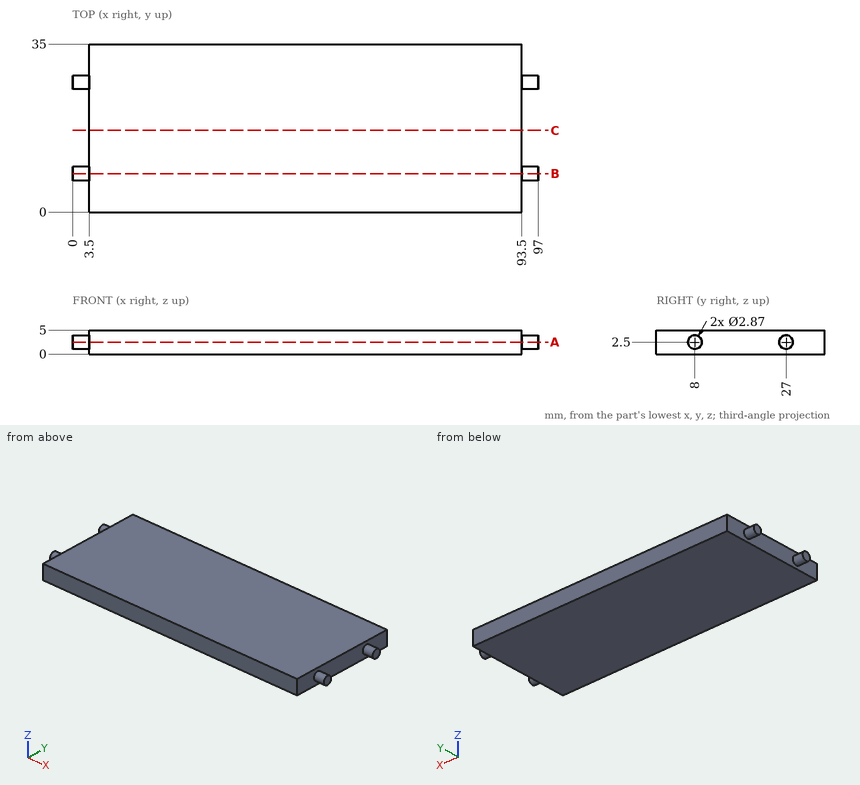
Geometry check sheet. Reference: drawing and pictorial views, mm from the part's lowest x, y, z. Give positions to 0.01 mm unless a question says otherwise; leave off trailing zeros. Write each loop counter-clockwise with the first axis right and the second up, starting at its lowest first coordinate (ties: lowest second). Pieces come first, ordered by that corner, then holes.
Item 1: Scan line: L1, parallel to X at y = 4, z = 2.2. Record every from-to range of solid material in increasing order.
Item 2: Cross-section at C-C (y = 17). Enter the section's corners in (x, z), and give its area (3 significant figures).
Item 3: Gauge pin test, flat ends, axial feed: pin 1 (3 mm diameter, centred on x = 64.5, z = 3, fed in from -Y); pin 2 (1.5 mm diameter, centred on y = 14, z = 1, fed in from +X); pin 3 (2.5 mm diameter, centred on y = 14.5, z = 3, fed in from -X). Record the tip position at first contact, or that the pin passes through.
Item 4: Cross-section at B-B (y = 8). Enter the section's corners in (x, z) (3 decimals), and give its area (3 significant figures).
Item 5: Cross-section at A-A (z = 2.5). Enter the section's corners in (x, y) (3 decimals).
Report:
1. L1: x = 3.5 to 93.5
2. outline: (3.5, 0) - (93.5, 0) - (93.5, 5) - (3.5, 5) - close
2. area: 450 mm2
3. pin 1: stops at y = 0
3. pin 2: stops at x = 93.5
3. pin 3: stops at x = 3.5
4. outline: (0, 1.065) - (3.5, 1.065) - (3.5, 0) - (93.5, 0) - (93.5, 1.065) - (97, 1.065) - (97, 3.935) - (93.5, 3.935) - (93.5, 5) - (3.5, 5) - (3.5, 3.935) - (0, 3.935) - close
4. area: 470 mm2
5. outline: (0, 6.565) - (3.5, 6.565) - (3.5, 0) - (93.5, 0) - (93.5, 6.565) - (97, 6.565) - (97, 9.435) - (93.5, 9.435) - (93.5, 25.565) - (97, 25.565) - (97, 28.435) - (93.5, 28.435) - (93.5, 35) - (3.5, 35) - (3.5, 28.435) - (0, 28.435) - (0, 25.565) - (3.5, 25.565) - (3.5, 9.435) - (0, 9.435) - close
